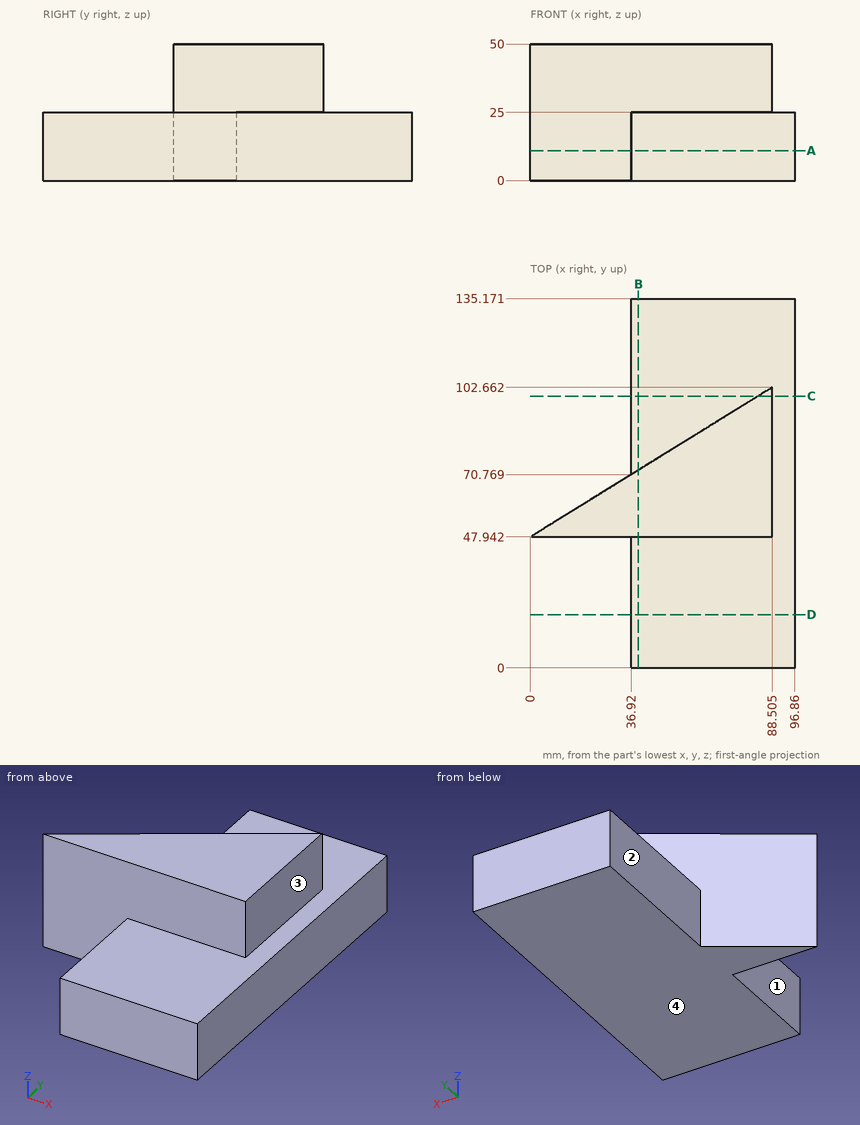
Design review of the part shown in the three views and the two pictorial views. Dimensions are in mm from the part's minimum x, y and z. A direction names the side the tool comes from. Round coordinates to 2 decimals unless told otherwise and drop trailing zeros. Loops run counter-clockwise (first coordinate to the right, second up) from the corner with the lowest first, then second, coordinate; pieces in that order, holes last. Notation, with made-up numbers: M -30,-19.5 L -8,-19.5 A16 ccw -8,-3.5 Z; hole C 17,-34.75 d11. An arc over 180 degrees is marked long. Write item = value, one per line.
Item 1: Insertion check: P1, Ø2, axis at y = 36.5, z = 12.5, coming from the -X side; P2, Ø1.5, axis at y = 73.5, z = 31, coming from the +X side (1 decimal); P3, Ø4, axis at x = 84, y = 57.5, coming from the -Z side; P4, Ø10, axis at y = 63.5, z = 27, coming from the -X side (1 decimal). Each pin has a flat end and moves straight along its axis. Give the tip position at first contact, or say it passes through.
Return value:
P1 = 36.92
P2 = 88.5
P3 = 0
P4 = 17.1
Item 2: Take a section at C-C on y = 99.5. Write out the cut boundary in (x, z) (1 decimal), then the cut area to 3 significant figures.
Return value:
outline = M 36.9,0 L 96.9,0 L 96.9,25 L 88.5,25 L 88.5,50 L 83.4,50 L 83.4,25 L 36.9,25 Z
area = 1,630 mm2
Item 3: Take a section at D-D on y = 19.5. Write out the cut boundary in (x, z), then the cut area to 3 significant figures.
Return value:
outline = M 36.92,0 L 96.86,0 L 96.86,25 L 36.92,25 Z
area = 1,500 mm2
Item 4: Take a section at A-A on z = 11. Write out the cut boundary in (x, y), then the cut area to 3 significant figures.
Return value:
outline = M 0,47.94 L 36.92,47.94 L 36.92,0 L 96.86,0 L 96.86,135.17 L 36.92,135.17 L 36.92,70.77 Z
area = 8,520 mm2
Item 5: Take a section at B-B on x = 39.5. Write out the cut boundary in (y, z).
Return value:
outline = M 0,0 L 135.17,0 L 135.17,25 L 72.36,25 L 72.36,50 L 47.94,50 L 47.94,25 L 0,25 Z
Item 6: For line 1 (Z direction, x = 88, y = 32.5); line 2 (X direction, y = 33.5, z = 7); line 3 (Y direction, x = 20, z = 21.5), list the stretches that pass through material, from the lowest coordinate up. Write a range as [from, to].
Return value:
line_1 = [0, 25]
line_2 = [36.92, 96.86]
line_3 = [47.94, 60.31]
Item 7: Machinability: for the marked faces 1, 2, 3 and 4, which of the approach directions +Z, -Z, +X, -X, +Y, -Y give a long, thin tool a straight path to every point of the face, cutting with its end or side? Answer none if there is none.
Return value:
face_1 = +Z, -Z, -X, -Y
face_2 = +Z, -Z, -X, +Y
face_3 = +Z, +X, +Y, -Y
face_4 = -Z, +X, -X, +Y, -Y
